Here's how the part is built. I have some questions about the finished solid (model axes, mm). A direction names the side the tool comes from. Give positions to 0.01 mm unless a question says otherwise; leave off trailing zeros. Write each loop counter-clockwise with the first axis right and the second up, starting at its lowest first coordinate (ties: lowest second). Pieces come first, ordered by that corner, then holes. Notation, with made-up numbers: (86, 87) - (131, 87) arc R36 ccw to (131, 123) - close; hole circle Ø9 at (27.5, 27). An arc over 180 degrees is marked (long way). One line per item, written item: value. Start each with the question number.
1) Imagine slicing it at A-A on x = -1. Write out the boundary of the cut face in (y, z) (1 decimal).
2) I'm going to push flat-ended pins straight in: P1, Ø5, axis at x = 24, y = -2.5, coming from the +Z side (3 decimals); P2, Ø2.5, axis at x = -4.5, z = -1.5, coming from the -Y side; P3, Ø4, axis at x = 37, y = -1, coming from the -Z side (3 decimals); P4, Ø2.5, axis at x = -4, z = 0.5, coming from the +Y side. Where does each tip first touch, or does it pass through?
3) We'd pull the mould along Y, two halves only. Please class faces 3 (the cylindrical face through (-2.13, -1.03, 4.65)), 4 (the flat face through (-4, 0.952, 0)), 5 (the flat face through (0, -2, 4)): +Y half, -Y half, draft (parallel to the pull), parting line (faces both ways), or undercut.
4) On a 3-axis mill with a long thin cutter (end or side, diameter ignored), from which of +Z, -Z, +X, -X, +Y, -Y can I reach the whole of each face in a straight line? I mean faces 1 (the flat face through (-4, -0.952, 0)), 2 (the cylindrical face through (34.1, -0.69, 3.1)). Say none if no direction works.
5) Please list where these lines run through material, in increasing order: L1, parallel to X at y = 0, z = 0; L2, parallel to X at y = 2, z = 4; L3, parallel to Z at x = 28.5, y = 1.25. Write a range as [from, to].
Autodesk Inventor part; units mm, degrees
ref_plane "IDS_WORKPLANE{1}" through (-5.4864, 0, 0) normal (1, 0, 0) x (0, 0, -1)
ref_plane "Work Plane2" through (41.275, 0, 0) normal (0, 0, -1) x (1, 0, 0)
ref_plane "YZ Plane" through (0, 0, 0) normal (1, 0, 0) x (0, 1, 0)
sketch "Sketch1" plane through (0, 0, 0) normal (0, 0, 1) x (1, 0, 0)
  line L0 (-5.4864, 0) -> (69.85, 0)
  line L1 (69.85, 0) -> (69.85, 3.175)
  line L2 (69.85, 3.175) -> (50.8, 3.175)
  line L3 (50.8, 3.175) -> (50.038, 3.175)
  line L4 (50.038, 3.175) -> (0, 3.175)
  line L5 (0, 3.175) -> (0, 4.7625)
  line L6 (-20.9299, 0) -> (84.98, 0)
  line L7 (0, -0.9693) -> (0, 5.8158)
  line L8 (0, 4.7625) -> (-4.2103, 4.7625)
  arc A0 (-4.2103, 4.7625) -> (-5.4864, 0) centre (4.0386, 0) ccw
  line L9 (50.8, 3.175) -> (0, 3.175) construction
  dimension "d0" = 69.85
  dimension "d1" = 19.05
  dimension "d2" = 0.762
  dimension "d3" = 5.4864
  dimension "d4" = 6.35
  dimension "d5" = 6.35
  dimension "d9" = 9.525
  dimension "d10" = 0
  dimension "d13" = 9.525
revolve "Body" add sketch "Sketch1" angle 360 about axis through (-5.4864, 0, 0) along (1, 0, 0)
ref_plane "IDS_WORKPLANE{1}" through (-5.4864, 0, 0) normal (1, 0, 0) x (0, 0, -1)
sketch "Sketch2" plane through (-5.4864, 0, 0) normal (1, 0, 0) x (0, 0, -1)
  circle A0 centre (0, 0) radius 4.7625
  line L0 (0, -6.6675) -> (0, 6.6675)
  line L1 (6.6675, 0) -> (-6.6675, 0)
  line L2 (-4.7625, 0.9525) -> (4.7625, 0.9525)
  line L3 (4.7625, 0.9525) -> (4.7625, -0.9525)
  line L4 (4.7625, -0.9525) -> (-4.7625, -0.9525)
  line L5 (-4.7625, -0.9525) -> (-4.7625, 0.9525)
  line L6 (-4.7625, 0) -> (4.7625, 0) construction
  line L7 (0, 0.9525) -> (0, -0.9525) construction
  dimension "d15" = 1.905
extrude "Slot" cut sketch "Sketch2" along normal blind 2.4638 contours L1 L0 L2 A0 | L3 L4 A0 | A0 L4 L0 L1 | A0 L2 L3 | L1 A0 L2 L0 | L0 L4 A0 L1 | L5 L2 A0 | A0 L4 L5
thread "Thread"
sketch "Sketch3" plane through (0, 0, 0) normal (0, 0, 1) x (1, 0, 0)
  line L0 (69.85, 0) -> (69.85, 3.175)
  line L1 (69.85, 3.175) -> (50.8, 3.175)
  line L2 (-5.4864, 0) -> (69.85, 0)
  arc A0 (69.85, 0) -> (68.9993, 3.175) centre (63.5, 0) ccw
  line L3 (69.85, -3.175) -> (69.85, 3.175)
  line L4 (68.9993, 3.175) -> (68.9993, 0)
  line L5 (68.9993, 0) -> (69.85, 0)
  dimension "d40" = 6.35
revolve "Fillet1" cut sketch "Sketch3" angle 360 about axis through (-5.4864, 0, 0) along (1, 0, 0) contours A0 L1 L0
chamfer "Chamfer" distance 0.635 angle 45 1 edges at (68.9993, -3.175, 0)
ref_plane "Work Plane2" through (41.275, 0, 0) normal (0, 0, -1) x (1, 0, 0)
fillet "Fillet4" radius 0.7874 1 edges at (0, -3.175, 0)
equation "\"d0\" = NLG"
equation "\"d1\" = GEL"
equation "\"d2\" = GAL"
equation "\"d3\" = KOH"
equation "\"d4\" = GD"
equation "\"d5\" = BDM"
equation "\"d9\" = KOD"
equation "\"d13\" = KR"
equation "\"d15\" = SBR"
equation "\"d16\" = STI"
equation "\"d40\" = GD"
equation "\"d46\" = R"
equation "\"d11\" = GEL"
equation "\"d43\" = 0.5 * RR"
equation "\"GD\" = NND"
equation "\"NLG\" = 69.85"
equation "\"GEL\" = 19.05"
equation "\"KOD\" = 9.525"
equation "\"KOH\" = 5.4864"
equation "\"GAL\" = 0.762"
equation "\"BDM\" = NND"
equation "\"SBR\" = 1.905"
equation "\"STI\" = 2.4638"
equation "\"KEWI\" = 0"
equation "\"KR\" = KOD"
equation "\"d14\" = -KOH"
equation "\"R\" = 0.7874"
equation "\"THREADDIA\" = 6.35"
equation "\"TOA\" = 30deg"
equation "\"KOH1\" = 4.3688"
equation "\"NND\" = 6.35"
equation "\"GD1\" = 4.8387"
equation "\"THREADDESC\" = 1.2345"
properties part number "ANSI B18.6.2 - 1/4-20 UNC - 2.75, SFHCSI" material "Steel, Mild"
Numbers:
1. outline: circle Ø9.5 at (0, 0)
2. P1: z = 3.175
2. P2: y = -4.75
2. P3: z = -3.175
2. P4: y = 4.76
3. face 3: parting line
3. face 4: undercut
3. face 5: draft
4. face 1: +Z, -Z, -X
4. face 2: +X
5. L1: [-3.02, 69.85]
5. L2: [-4.37, 0]
5. L3: [-2.92, 2.92]
